Read the model definition and answer for the solid it produces. Units are mm, in the model's axes. Face numbers are marked on the shaded views. A direction names the side the tool comes from. Give positions to 0.01 mm unless a question says otherwise; leave off trailing zeros. Order: outer loops, then holes, each group sorted by start corner. A loop starts at its lowest first (then second) coordinate and runs counter-clockwise, first axis right, second up. Notation, with made-up numbers: (-22, -30) - (34, -30) arc R22 ccw to (34, -9) - close; hole circle Ø11 at (28, 65.5). An arc over 180 degrees is marked (long way). Return JSON: item names as keys, results as strings.
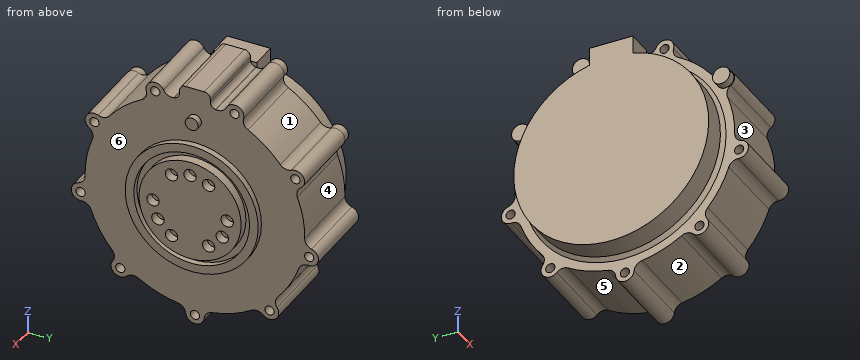
```python
from build123d import *

# Parameters (mm, degrees)
SKETCH009_R        = 16.5
SKETCH009_R_2      = 2
PAD006_DEPTH       = 3
SKETCH010_R        = 1.5
PAD007_DEPTH       = 25
POLARPATTERN_COUNT = 9
PAD008_DEPTH       = 25
SKETCH012_R        = 21.5
SKETCH012_R_2      = 18.7
SKETCH012_R_3      = 2.1
PAD009_DEPTH       = 2
PAD010_DEPTH       = 8.5
SKETCH014_R        = 2.8
PAD011_DEPTH       = 2.6
CHAMFER_SIZE       = 1.2


with BuildPart() as part:
    # Sketch009 → Pad006 (new body)
    with BuildSketch(Plane.YZ):
        Circle(SKETCH009_R)
        with Locations((0, 12)):
            Circle(SKETCH009_R_2, mode=Mode.SUBTRACT)
        with Locations((-6, 10.392305)):
            Circle(SKETCH009_R_2, mode=Mode.SUBTRACT)
        with Locations((6, 10.392305)):
            Circle(SKETCH009_R_2, mode=Mode.SUBTRACT)
        with Locations((12, 0)):
            Circle(SKETCH009_R_2, mode=Mode.SUBTRACT)
        with Locations((10.392305, -6)):
            Circle(SKETCH009_R_2, mode=Mode.SUBTRACT)
        with Locations((6, -10.392305)):
            Circle(SKETCH009_R_2, mode=Mode.SUBTRACT)
        with Locations((-6, -10.392305)):
            Circle(SKETCH009_R_2, mode=Mode.SUBTRACT)
        with Locations((-10.392305, -6)):
            Circle(SKETCH009_R_2, mode=Mode.SUBTRACT)
        with Locations((-12, 0)):
            Circle(SKETCH009_R_2, mode=Mode.SUBTRACT)
    extrude(amount=PAD006_DEPTH)

    # Sketch010 → Pad007 (join)
    with BuildSketch(Plane.YZ):
        with BuildLine():
            ThreePointArc((5.510568, -35.069697), (0, 35.5), (-5.510568, -35.069697))
            ThreePointArc((-2.988125, -37.766667), (-3.785221, -35.984091), (-5.510568, -35.069697))
            ThreePointArc((-2.988125, -37.766667), (0, -40.5), (2.988125, -37.766667))
            ThreePointArc((5.510568, -35.069697), (3.785221, -35.984091), (2.988125, -37.766667))
        make_face()
        with Locations((0, -37.5)):
            Circle(SKETCH010_R, mode=Mode.SUBTRACT)
    pad007 = extrude(amount=-PAD007_DEPTH)

    # PolarPattern: Pad007 ×9 about axis
    polarpattern_axis = Axis((0, 0, 0), (1, 0, 0))
    for i in range(1, POLARPATTERN_COUNT):
        add(pad007.rotate(polarpattern_axis, i * 360 / POLARPATTERN_COUNT))

    # Sketch011 → Pad008 (join)
    with BuildSketch(Plane.YZ):
        with BuildLine():
            ThreePointArc((-6.626667, 34.876027), (-5.459437, 35.565466), (-5, 36.840874))
            Line((-5, 37.840874), (-5, 36.840874))
            ThreePointArc((-3, 39.840874), (-4.414214, 39.255088), (-5, 37.840874))
            Line((-3, 39.840874), (3, 39.840874))
            ThreePointArc((5, 37.840874), (4.414214, 39.255088), (3, 39.840874))
            Line((5, 37.840874), (5, 36.840874))
            ThreePointArc((5, 36.840874), (5.459437, 35.565466), (6.626667, 34.876027))
            ThreePointArc((6.626667, 34.876027), (0, 35.5), (-6.626667, 34.876027))
        make_face()
    extrude(amount=-PAD008_DEPTH)

    # Sketch012 → Pad009 (join)
    with BuildSketch(Plane.YZ):
        Circle(SKETCH012_R)
        Circle(SKETCH012_R_2, mode=Mode.SUBTRACT)
        with Locations((0, 29)):
            Circle(SKETCH012_R_3)
    extrude(amount=PAD009_DEPTH)

    # Sketch013 → Pad010 (join)
    with BuildSketch(Plane.YZ.offset(-25)):
        with BuildLine():
            ThreePointArc((-7, 30.712375), (0, -31.5), (7, 30.712375))
            Line((7, 36.5), (7, 30.712375))
            Line((-7, 36.5), (7, 36.5))
            Line((-7, 30.712375), (-7, 36.5))
        make_face()
    extrude(amount=-PAD010_DEPTH)

    # Sketch014 → Pad011 (join)
    with BuildSketch(Plane.YZ.offset(-25)):
        with Locations((12.825755, 35.238473)):
            Circle(SKETCH014_R)
        with Locations((32.475953, 18.75)):
            Circle(SKETCH014_R)
        with Locations((-32.475953, 18.75)):
            Circle(SKETCH014_R)
    extrude(amount=-PAD011_DEPTH)

    # Chamfer
    chamfer_edges = [part.edges().sort_by_distance(p)[0] for p in [
        (-25, 0, -31.5),
    ]]
    chamfer(chamfer_edges, length=CHAMFER_SIZE)


with BuildPart() as part_1:
    # Body009 placement: moved
    add(part.part.moved(Location((-38.8, 0, 55.540956))))


with BuildPart() as part_2:
    # Clone003 placement: moved
    add(part_1.part.moved(Location((38.8, 0, -55.540956))))


with BuildPart() as part_3:
    # Body010 placement: moved
    add(part_2.part.moved(Location((47, 0, 107))))


solid = part_3.part
```
Q1. A cutting plane is placed at D-D (x = 17.5). Write down the section's boundary in (y, z), and give its area (3 significant figures).
Values:
{"outline": "(-7, 137.71) arc R31.5 ccw (long way) to (7, 137.71) - (7, 143.5) - (-7, 143.5) - close", "area": "3,190 mm²"}
Q2. Determine the mould class of the marked faces 1, 2 and 3 for opening direction Y: released by +Y, released by -Y, zero draft, split by the parting line, or undercut.
Values:
{"face 1": "released by +Y", "face 2": "undercut", "face 3": "released by -Y"}
Q3. A cutting plane is placed at B-B (x = 34). Give the number of separate pieces and of enclosed holes in the cut face, and give its area (3 significant figures).
Values:
{"separate pieces": "1", "enclosed holes": "9", "area": "4,200 mm²"}
Q4. Consider L1, parallel to Y at x = 38, z = 125 (3 decimals); L2, parallel to Z at x = 48, y = -0.5; L3, parallel to X at y = 34, z = 123.5. Determine where each line is inside the solid, lowest interval first.
Values:
{"L1": "y = -35.381 to -33.775, -31.177 to 31.177, 33.775 to 35.381", "L2": "z = 85.51 to 88.31, 90.51 to 117.06, 120.94 to 123.49, 125.69 to 128.49, 133.96 to 138.04", "L3": "x = 19.4 to 47"}
Q5. Given pin 1 (5 mm diameter, centred on y = 12.83, z = 142.24, fed in from -X); pin 2 (4 mm diameter, centred on y = -36.93, z = 100.49, fed in from -X); pin 3 (1 mm diameter, centred on x = 28.5, z = 80.5, fed in from +Y), each flat-ended and moving along its own axis, determine where each tip first touches the part or whether it passes through.
Values:
{"pin 1": "stops at x = 19.4", "pin 2": "stops at x = 22", "pin 3": "stops at y = 26.56"}
Q6. For the marked faces 4, 5 and 6, determine the directions among +Z, -Z, +X, -X, +Y, -Y from which every point of the face is accessible in a straight line to the end or side of a thin tool.
Values:
{"face 4": "+X, -X, +Y", "face 5": "-Z, +X, -X", "face 6": "+X"}
